Verification items for this drawing (mm, ordinates from the low corner). A direction names the side the tool comes from. Coordinates: 2 decimals unless noted, no trailing zeros. Order: outer loops, then holes, each group sorted by start corner. A loop starts at its lowest first (then second) coordinate and runs counter-clockwise, first axis right, second up. Notation, with made-up numbers: (-4.5, 59) -> (48.5, 59) arc R17 ccw to (48.5, 83) -> close; hole circle Ø2 at (45.25, 13). An arc over 180 degrees is marked (long way). Answer in a Markdown table with one row per item. Add a question column.
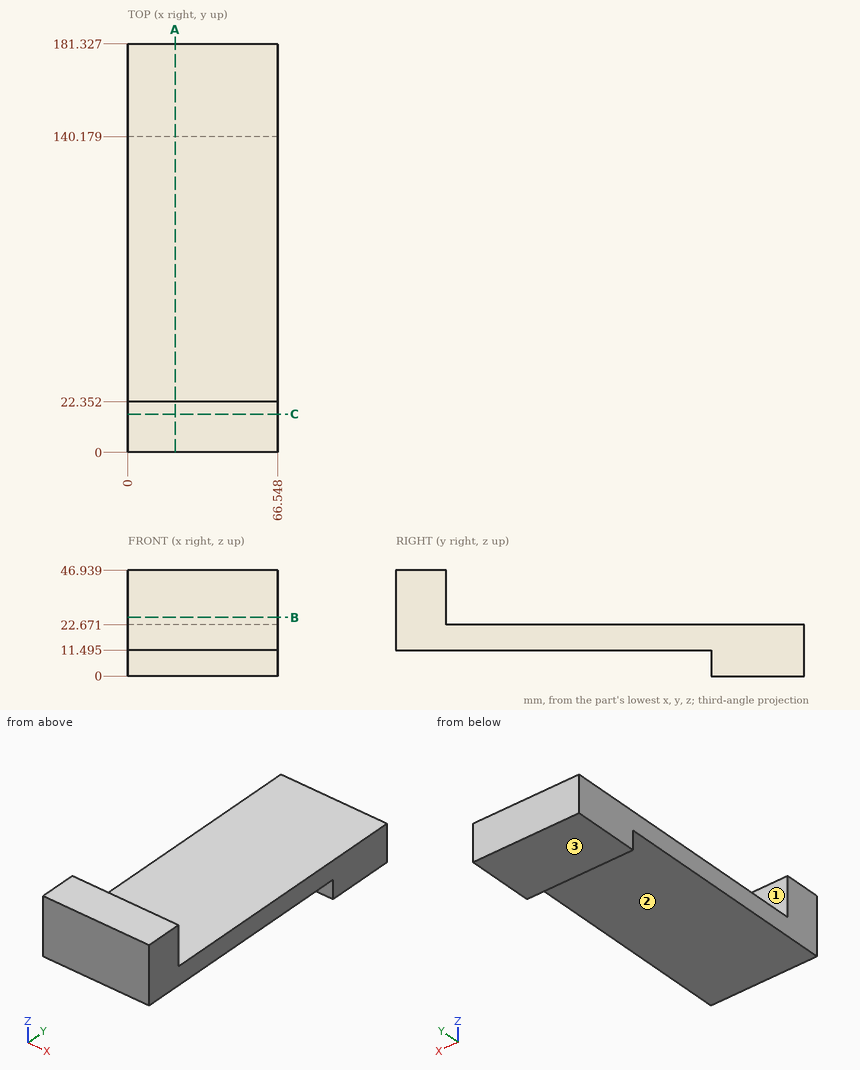
(1) Cross-section at A-A (x = 21). Enter the section's corners in (y, z) (1 decimal).
(2) Scan lines: line 1 along Y through (x, z) = (48.5, 23); line 2 along Z through (x, y) = (63, 153); line 3 along Z through (x, y) = (27.5, 99.5) (1 decimal). Record each from-to range of solid material in increasing order.
(3) Access from +Z, -Z, +X, -X, +Y, -Y to the whole of each face (thin tool, end or side, straight path). Record for the marked faces 1, 2 and 3.
(4) Go/stop test with flat-tipped pins: P1, Ø20, axis at x = 36, y = 85, coming from the -Z side (1 decimal); P2, Ø20, axis at x = 47, y = 84.5, coming from the +Z side; P3, Ø8, axis at x = 59.5, z = 12.5, coming from the -Y side; P4, Ø3, axis at x = 52.5, z = 27, coming from the +Y side. Record where each tip stops, or that it passes through.
(5) Cross-section at C-C (y = 17). Enter the section's corners in (x, z) (1 decimal).
(6) Cross-section at B-B (z = 26). Enter the section's corners in (x, y).
Checks:
| question | item | result |
|---|---|---|
| 1 | outline | (0, 11.5) -> (140.2, 11.5) -> (140.2, 0) -> (181.3, 0) -> (181.3, 22.7) -> (22.4, 22.7) -> (22.4, 46.9) -> (0, 46.9) -> close |
| 2 | line 1 | 0 to 22.35 |
| 2 | line 2 | 0 to 22.67 |
| 2 | line 3 | 11.5 to 22.7 |
| 3 | face 1 | +Z, +X, -X, +Y |
| 3 | face 2 | -Z, +X, -X, -Y |
| 3 | face 3 | -Z, +X, -X, +Y, -Y |
| 4 | P1 | z = 11.5 |
| 4 | P2 | z = 22.67 |
| 4 | P3 | y = 0 |
| 4 | P4 | y = 22.35 |
| 5 | outline | (0, 11.5) -> (66.5, 11.5) -> (66.5, 46.9) -> (0, 46.9) -> close |
| 6 | outline | (0, 0) -> (66.55, 0) -> (66.55, 22.35) -> (0, 22.35) -> close |
